```python
from build123d import *

# Parameters (mm, degrees)
F1_DEPTH       = 19.05
F2_R           = 6.35
F3_SIZE2       = 50.8
F3_SIZE        = 50.8
F4_R           = 3.175
F5_DEPTH       = 25.4
F6_D           = 12.7
F6_DEPTH       = 12.7
F6_TIP         = 3.8154649308
F7_D           = 9.525
F7_DEPTH       = 25.4
F7_CBORE_D     = 12.7
F7_CBORE_DEPTH = 12.7
F7_TIP         = 2.8615986981


# Not quite as in the source:
# - a feature names something its author has since deleted; it is built from what else it names


with BuildPart() as f1:
    # F0 (on Front) → F1 (new body)
    with BuildSketch(Plane.XZ):
        Polygon((-61.5315027535, 184.1499997646), (-61.5315027535, -19.0500002354), (-23.4315027535, -19.0500002354), (-23.4315027535, 6.3499997646), (205.1684972465, 6.3499997646), (205.1684972465, -19.0500002354), (243.2684972465, -19.0500002354), (243.2684972465, 184.1499997646), align=None)
    extrude(amount=F1_DEPTH)

    # F2
    f2_edges = [f1.edges().sort_by_distance(p)[0] for p in [
        (-23.431503, -9.525, 6.35),
        (-61.531503, -9.525, -19.05),
        (243.268497, -9.525, -19.05),
        (205.168497, -9.525, -19.05),
        (205.168497, -9.525, 6.35),
        (-23.431503, -9.525, -19.05),
    ]]
    fillet(f2_edges, radius=F2_R)

    # F3
    f3_edges = [f1.edges().sort_by_distance(p)[0] for p in [
        (243.268497, -9.525, 184.15),
        (-61.531503, -9.525, 184.15),
    ]]
    chamfer(f3_edges, length=F3_SIZE, length2=F3_SIZE2)

    # F4 (on face) → F5 (cut)
    with BuildSketch(Plane.XZ.offset(19.05)):
        with Locations((59.1184972465, 19.0499997646)):
            Circle(F4_R)
        with Locations((122.6184972465, 19.0499997646)):
            Circle(F4_R)
    extrude(amount=-F5_DEPTH, mode=Mode.SUBTRACT)

    # F6
    with Locations(Plane.XZ.offset(19.05)):
        with Locations((-36.1315027535, 115.1381997646), (217.8684972465, 115.1381997646)):
            Hole(F6_D / 2, depth=F6_DEPTH)
            with Locations((0, 0, -(F6_DEPTH + F6_TIP / 2))):  # 118° drill point
                Cone(0, F6_D / 2, F6_TIP, mode=Mode.SUBTRACT)

    # F7
    with Locations(Plane.XZ.offset(19.05)):
        with Locations((-42.4815027535, 76.1999997646), (-42.4815027535, -2.354e-07), (224.2184972465, -2.354e-07), (224.2184972465, 76.1999997646)):
            CounterBoreHole(F7_D / 2, F7_CBORE_D / 2, F7_CBORE_DEPTH, depth=F7_DEPTH)
            with Locations((0, 0, -(F7_DEPTH + F7_TIP / 2))):  # 118° drill point
                Cone(0, F7_D / 2, F7_TIP, mode=Mode.SUBTRACT)


solid = f1.part
```
Source: CAD feature listing. Evaluate the final solid. Frame: model axes, mm. A direction names the side the tool comes from. Round coordinates to 2 decimals unless told otherwise and drop trailing zeros. Order: outer loops, then holes, each group sorted by start corner. A loop starts at its lowest first (then second) coordinate and runs counter-clockwise, first axis right, second up. Notation, with made-up numbers: (82, 18.5) -> (95, 18.5) arc R20 ccw to (95, 50.5) -> close; hole circle Ø11 at (76, 61.5). An arc over 180 degrees is marked (long way). One line per item, written item: value. Start each with the question number.
Q1. Draft query along X for faces 1 (the cylindrical face through (241.4, -9.7, -17.2)), 2 (the flat face through (-23.432, -9, -6)), 3 (the flat face through (-61.532, -9, 61)), 4 (the cylindrical face through (-47.162, -12.789, 80.492)). Return one class per face: pulls with the +X half, pulls with the -X half, needs draft (parallel to the pull), parting line crosses it, or undercut.
Q2. Section query A-A (z = 19.05). Return the cut outline in (x, y), plus the area to 3 significant figures.
Q3. Material intervals for probe 1 along X at (y, z) = (-12.75, 0); probe 2 along X at (y, z) = (-4.75, 19.05); probe 3 along X at (y, z) = (-9.75, 76.2), sorted ascending.
Q4. Access query for faces 5 (the cylindrical face through (217.875, -12.789, 76.479)), 6 (the cylindrical face through (-25.3, -9.7, -17.2)), 7 (the flat face through (-43, -9, -19.05)). Directions: +Z, -Z, +X, -X, +Y, -Y. A direction counts if a zero-diameter tool reaches every point of the face in a straight line with its end or side. Return the directions, or none.
Q5. Section query B-B (z = 76.2). Return the cut outline in (x, y).
Q6. Pin query (flat end, axial travel): pin 1 (11.5 mm diameter, centred on x = -36.13, z = 115.14, fed in from -Y); pin 2 (9.5 mm diameter, centred on x = 84, y = -5, fed in from -Z). Return the tip coordinate at first contact, or that it passes through.
Findings below:
1. face 1: pulls with the +X half
1. face 2: undercut
1. face 3: pulls with the -X half
1. face 4: undercut
2. outline: (-61.53, -19.05) -> (55.94, -19.05) -> (55.94, 0) -> (-61.53, 0) -> close; (62.29, -19.05) -> (119.44, -19.05) -> (119.44, 0) -> (62.29, 0) -> close; (125.79, -19.05) -> (243.27, -19.05) -> (243.27, 0) -> (125.79, 0) -> close
2. area: 5,560 mm²
3. probe 1: -61.53 to -48.83, -36.13 to -23.43, 205.17 to 217.87, 230.57 to 243.27
3. probe 2: -61.53 to 55.94, 62.29 to 119.44, 125.79 to 243.27
3. probe 3: -61.53 to -48.83, -36.13 to 217.87, 230.57 to 243.27
4. face 5: -Y
4. face 6: -Z, +Y, -Y
4. face 7: -Z, +X, -X, +Y, -Y
5. outline: (-61.53, -19.05) -> (-48.83, -19.05) -> (-48.83, -6.35) -> (-47.24, -6.35) -> (-47.24, 0) -> (-61.53, 0) -> close; (-37.72, -6.35) -> (-36.13, -6.35) -> (-36.13, -19.05) -> (217.87, -19.05) -> (217.87, -6.35) -> (219.46, -6.35) -> (219.46, 0) -> (-37.72, 0) -> close; (228.98, -6.35) -> (230.57, -6.35) -> (230.57, -19.05) -> (243.27, -19.05) -> (243.27, 0) -> (228.98, 0) -> close
6. pin 1: y = -5.99
6. pin 2: z = 6.35
